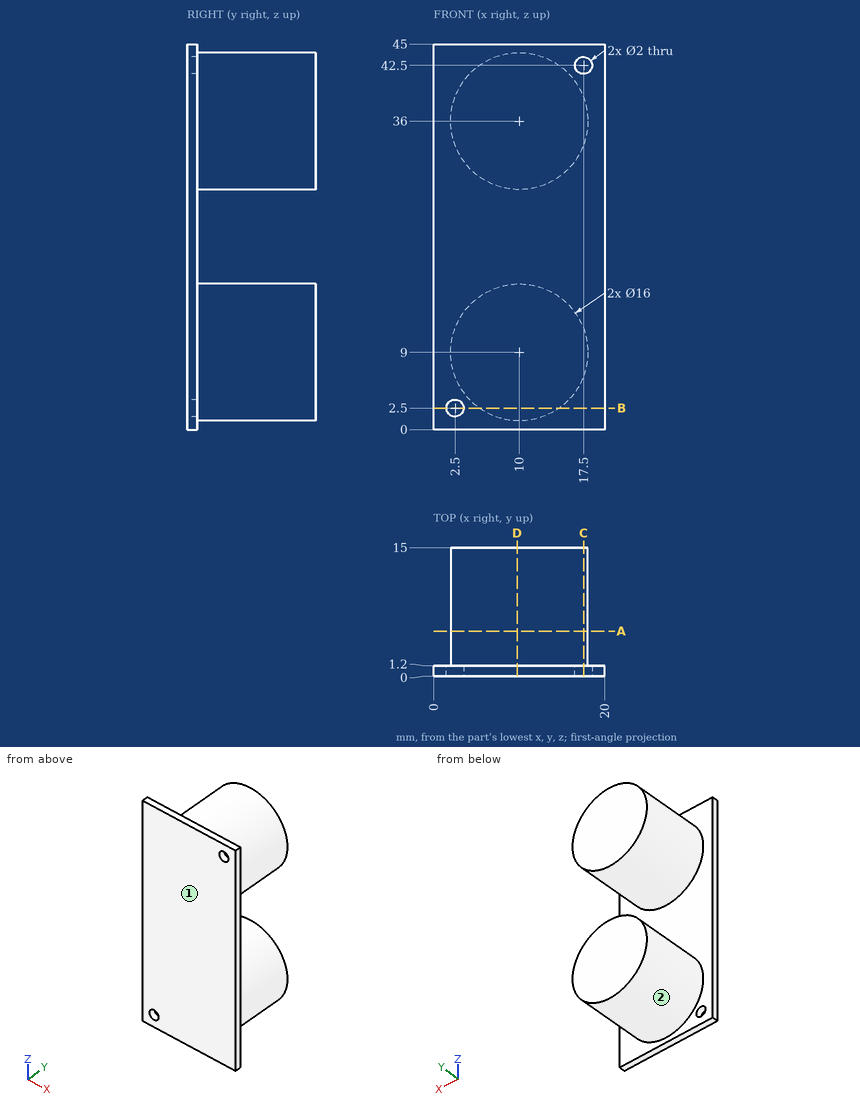
Here's the drawing with two shaded views (mm, measured from the low corner). I have some questions. A direction names the side the tool comes from. Round coordinates to 2 decimals unless told otherwise and drop trailing zeros. Loops run counter-clockwise (first coordinate to the right, second up) from the corner with the lowest first, then second, coordinate; pieces in that order, holes last. Notation, with made-up numbers: M 13.25,-23.75 L 44.25,-23.75 A11 ccw 44.25,-16.75 Z; hole C 37.5,15 d4. An arc over 180 degrees is marked long. Answer as a JSON object with one key per item and string values. Group by question number.
Q1. On a 3-axis mill with a long thin cutter (end or side, diameter ignored), from which of +Z, -Z, +X, -X, +Y, -Y can I reach the whole of each face in a straight line? I mean the marked faces 1 and 2. Say none if no direction works.
Q2. Imagine slicing it at D-D, the plane x = 9.75. Please give me the cut outline in (y, z), then the cut area to 3 significant figures.
Q3. Imagine slicing it at C-C, the plane x = 17.5. Please give me the cut outline in (y, z), then the cut area to 3 significant figures.
Q4. Please list where these lines run through material, in increasing order: L1, parallel to Z at x = 2.5, y = 0.2; L2, parallel to Y at x = 1.5, z = 23; L3, parallel to Z at x = 3.25, y = 9.5.
Q5. Imagine slicing it at B-B, the plane z = 2.5. Please give me the cut outline in (x, y), then the cut area to 3 significant figures.
Q6. Will these pins go through, and if not, where does the flat tip stop? pin 1 (1 mm diameter, centred on x = 9.5, z = 23, fed in from +Y); pin 2 (4 mm diameter, centred on x = 3, y = 12, fed in from +Z) (3 decimals).
Q7. Imagine slicing it at A-A, the plane y = 5.25. Please give me the cut outline in (x, z), then the cut area to 3 significant figures.
Findings:
{
 "1": {"face 1": "+Z, -Z, +X, -X, -Y", "face 2": "+Y"},
 "2": {"outline": "M 0,0 L 1.2,0 L 1.2,1 L 15,1 L 15,17 L 1.2,17 L 1.2,28 L 15,28 L 15,44 L 1.2,44 L 1.2,45 L 0,45 Z", "area": "495 mm2"},
 "3": {"outline": "M 0,0 L 1.2,0 L 1.2,6.22 L 15,6.22 L 15,11.78 L 1.2,11.78 L 1.2,33.22 L 15,33.22 L 15,38.78 L 1.2,38.78 L 1.2,41.5 L 0,41.5 Z; M 0,43.5 L 1.2,43.5 L 1.2,45 L 0,45 Z", "area": "205 mm2"},
 "4": {"L1": "z = 0 to 1.5, 3.5 to 45", "L2": "y = 0 to 1.2", "L3": "z = 4.71 to 13.29, 31.71 to 40.29"},
 "5": {"outline": "M 0,0 L 1.5,0 L 1.5,1.2 L 0,1.2 Z; M 3.5,0 L 20,0 L 20,1.2 L 14.66,1.2 L 14.66,15 L 5.34,15 L 5.34,1.2 L 3.5,1.2 Z", "area": "150 mm2"},
 "6": {"pin 1": "stops at y = 1.2", "pin 2": "stops at z = 42.245"},
 "7": {"outline": "C 10,9 d16; C 10,36 d16", "area": "402 mm2"}
}
